from build123d import *

# Parameters (mm, degrees)
F0_W      = 2057.4
F0_H      = 1143
F1_DEPTH  = 19.05
F3_DEPTH  = 50.8
F5_DEPTH  = 50.8
F7_DEPTH  = 50.8
F10_DEPTH = 50.8
F12_DEPTH = 50.8
F14_DEPTH = 50.8
F16_DEPTH = 50.8
F18_DEPTH = 50.8


with BuildPart() as f1:
    # F0 (on Top) → F1 (new body)
    with BuildSketch(Plane.XY):
        Polygon((1066.8, 609.6), (0, 609.6), (-1066.8, 609.6), (-1066.8, -609.6), (-1028.7, -609.6), (1066.8, -609.6), align=None)
        Rectangle(F0_W, F0_H, mode=Mode.SUBTRACT)
        Rectangle(F0_W, F0_H)
    extrude(amount=F1_DEPTH)

    # F2 (on face) → F3 (join)
    with BuildSketch(Plane(origin=(0, 0, 0), x_dir=(1, 0, 0), z_dir=(0, 0, -1))):
        Polygon((-914.4, -457.2), (0, -457.2), (914.4, -457.2), (914.4, 457.2), (0, 457.2), (-914.4, 457.2), align=None)
        Polygon((895.35, -438.15), (0, -438.15), (-895.35, -438.15), (-895.35, 438.15), (0, 438.15), (895.35, 438.15), align=None, mode=Mode.SUBTRACT)
    extrude(amount=F3_DEPTH)

    # F4 (on face) → F5 (join)
    with BuildSketch(Plane(origin=(0, -438.15, 0), x_dir=(-1, 0, 0), z_dir=(0, 1, 0))):
        with BuildLine():
            Line((895.35, -762), (895.35, 0))
            Line((895.35, 0), (742.95, 0))
            Line((742.95, 0), (615.95, 0))
            ThreePointArc((615.95, 0), (705.7525612107, -37.1974387893), (742.95, -127))
            ThreePointArc((742.95, -127), (763.4615182258, -201.0530890645), (819.15, -254))
            ThreePointArc((819.15, -254), (837.8461266285, -276.4019366858), (844.55, -304.8))
            Line((844.55, -304.8), (844.55, -762))
            Line((844.55, -762), (895.35, -762))
        make_face()
    extrude(amount=F5_DEPTH)

    # F6 (on face) → F7 (join)
    with BuildSketch(Plane.XZ.offset(-438.15)):
        with BuildLine():
            Line((-742.95, 0), (-895.35, 0))
            Line((-895.35, 0), (-895.35, -127))
            Line((-895.35, -127), (-895.35, -203.2))
            Line((-895.35, -203.2), (-895.35, -762))
            Line((-895.35, -762), (-844.55, -762))
            Line((-844.55, -762), (-844.55, -304.8))
            ThreePointArc((-844.55, -304.8), (-837.8461266285, -276.4019366858), (-819.15, -254))
            ThreePointArc((-819.15, -254), (-760.8906614316, -202.595603141), (-742.95, -127))
            ThreePointArc((-742.95, -127), (-705.7525612107, -37.1974387893), (-615.95, 0))
            Line((-615.95, 0), (-742.95, 0))
        make_face()
    extrude(amount=F7_DEPTH)

    # F8: F1 across plane


with BuildPart() as f1_1:
    add(f1.part)
    add(f1.part.mirror(Plane.YZ))

    # F9 (on face) → F10 (join)
    with BuildSketch(Plane.XZ.offset(438.15)):
        with BuildLine():
            Line((-844.55, -558.8), (-844.55, -762))
            ThreePointArc((-844.55, -762), (0, -642.6582759858), (844.55, -762))
            Line((844.55, -762), (844.55, -558.8))
            Line((844.55, -558.8), (-844.55, -558.8))
        make_face()
    extrude(amount=-F10_DEPTH)

    # F11 (on face) → F12 (join)
    with BuildSketch(Plane(origin=(0, 438.15, 0), x_dir=(-1, 0, 0), z_dir=(0, 1, 0))):
        with BuildLine():
            ThreePointArc((-844.55, -762), (0, -642.6582759858), (844.55, -762))
            Line((844.55, -762), (844.55, -558.8))
            Line((844.55, -558.8), (-844.55, -558.8))
            Line((-844.55, -558.8), (-844.55, -762))
        make_face()
    extrude(amount=-F12_DEPTH)

    # F13 (on face) → F14 (join)
    with BuildSketch(Plane.YZ.offset(-895.35)):
        with BuildLine():
            Line((-387.35, -560.2836336464), (-387.35, -762))
            ThreePointArc((-387.35, -762), (0, -644.1417336464), (387.35, -762))
            Line((387.35, -762), (387.35, -560.2836336464))
            Line((387.35, -560.2836336464), (-387.35, -560.2836336464))
        make_face()
    extrude(amount=F14_DEPTH)

    # F15 (on face) → F16 (join)
    with BuildSketch(Plane(origin=(895.35, 0, 0), x_dir=(0, -1, 0), z_dir=(-1, 0, 0))):
        with BuildLine():
            Line((-387.35, -558.8), (-387.35, -762))
            ThreePointArc((-387.35, -762), (0, -642.6581), (387.35, -762))
            Line((387.35, -762), (387.35, -558.8))
            Line((387.35, -558.8), (-387.35, -558.8))
        make_face()
    extrude(amount=F16_DEPTH)

    # F17 (on face) → F18 (join)
    with BuildSketch(Plane.YZ.offset(-895.35)):
        with BuildLine():
            Line((387.35, -304.8), (387.35, 0))
            Line((387.35, 0), (158.75, 0))
            ThreePointArc((158.75, 0), (248.5525612107, -37.1974387893), (285.75, -127))
            ThreePointArc((285.75, -127), (306.2615182258, -201.0530890645), (361.95, -254))
            ThreePointArc((361.95, -254), (380.6461266285, -276.4019366858), (387.35, -304.8))
        make_face()
        with BuildLine():
            Line((-387.35, 0), (-387.35, -304.8))
            ThreePointArc((-387.35, -304.8), (-380.6461266285, -276.4019366858), (-361.95, -254))
            ThreePointArc((-361.95, -254), (-306.2615182258, -201.0530890645), (-285.75, -127))
            ThreePointArc((-285.75, -127), (-248.5525612107, -37.1974387893), (-158.75, 0))
            Line((-158.75, 0), (-387.35, 0))
        make_face()
    extrude(amount=F18_DEPTH)

    # F19: F1 across plane


with BuildPart() as f1_2:
    add(f1_1.part)
    add(f1_1.part.mirror(Plane.YZ))


solid = f1_2.part
The model under review builds one solid part; all positions refer to its coordinate system, in mm. A direction names the side the tool comes from. Round coordinates to 2 decimals unless told otherwise and drop trailing zeros. Order: outer loops, then holes, each group sorted by start corner. A loop starts at its lowest first (then second) coordinate and runs counter-clockwise, first axis right, second up. Notation, with made-up numbers: (-36, -16) -> (4, -16) arc R14 ccw to (4, -9) -> close; hole circle Ø11 at (60, 6). An arc over 180 degrees is marked (long way). Return JSON: item names as keys, results as strings.
1. Take a section at D-D (x = 499). Write out the cut boundary in (y, z), then the cut area to 3 significant figures.
Answer block:
{"outline": "(-609.6, 0) -> (-457.2, 0) -> (-457.2, -50.8) -> (-438.15, -50.8) -> (-438.15, 0) -> (438.15, 0) -> (438.15, -50.8) -> (457.2, -50.8) -> (457.2, 0) -> (609.6, 0) -> (609.6, 19.05) -> (-609.6, 19.05) -> close; (-438.15, -683.78) -> (-387.35, -683.78) -> (-387.35, -558.8) -> (-438.15, -558.8) -> close; (387.35, -683.78) -> (438.15, -683.78) -> (438.15, -558.8) -> (387.35, -558.8) -> close", "area": "37,900 mm²"}
2. Take a section at C-C (y = -229.5). Write out the cut boundary in (x, z).
Answer block:
{"outline": "(-1066.8, 0) -> (-914.4, 0) -> (-914.4, -50.8) -> (-895.35, -50.8) -> (-895.35, -21.53) -> (-844.55, -21.53) -> (-844.55, 0) -> (844.55, 0) -> (844.55, -21.53) -> (895.35, -21.53) -> (895.35, -50.8) -> (914.4, -50.8) -> (914.4, 0) -> (1066.8, 0) -> (1066.8, 19.05) -> (-1066.8, 19.05) -> close; (-895.35, -683.1) -> (-844.55, -683.1) -> (-844.55, -558.8) -> (-895.35, -558.8) -> close; (844.55, -683.1) -> (895.35, -683.1) -> (895.35, -558.8) -> (844.55, -558.8) -> close"}
3. For faces 1 (the face through (870, -5, -558.8)), 2 (the face through (12, 387.35, -614)), 3 (the face through (-706.735, 413.106, -38.19)), list the 3-axis set-ups (+Z, -Z, +X, -X, +Y, -Y) from which the entire face can be reached by the end or side of a thin tool; tool diameter is ignored.
Answer block:
{"face 1": "+X, -X", "face 2": "-Z", "face 3": "none"}
4. The part is to be moulded in two halves that separate along X. For faces 4 (the face through (-837.66, -413.11, -276.03)), 5 (the face through (-914.4, -6, -25)), 6 (the face through (-870.31, 380.46, -276.03)), 7 (the face through (-13, 6, 0)), say which applies: +X half, -X half, draft (parallel to the pull), parting line (faces both ways), or undercut.
Answer block:
{"face 4": "undercut", "face 5": "-X half", "face 6": "draft", "face 7": "undercut"}
5. Insertion check: P1, Ø15, axis at x = -286, z = -20, coming from the -Y side; P2, Ø6, axis at x = -466.5, y = 95, coming from the -Z side; P3, Ø15, axis at y = 402.5, z = -486, coming from the +X side. Each pin has a flat end and moves straight along its axis. Give the tip position at first contact, or say it passes through.
Answer block:
{"P1": "stops at y = -457.2", "P2": "stops at z = 0", "P3": "stops at x = 895.35"}
6. Take a section at A-A (x = -435.5). Write out the cut boundary in (y, z).
Answer block:
{"outline": "(-609.6, 0) -> (-457.2, 0) -> (-457.2, -50.8) -> (-438.15, -50.8) -> (-438.15, 0) -> (438.15, 0) -> (438.15, -50.8) -> (457.2, -50.8) -> (457.2, 0) -> (609.6, 0) -> (609.6, 19.05) -> (-609.6, 19.05) -> close; (-438.15, -673.93) -> (-387.35, -673.93) -> (-387.35, -558.8) -> (-438.15, -558.8) -> close; (387.35, -673.93) -> (438.15, -673.93) -> (438.15, -558.8) -> (387.35, -558.8) -> close"}
7. Take a section at B-B (z = -192.5). Write out the cut boundary in (x, y), then the cut area to 3 significant figures.
Answer block:
{"outline": "(-895.35, -438.15) -> (-758.72, -438.15) -> (-758.72, -387.35) -> (-844.55, -387.35) -> (-844.55, -301.52) -> (-895.35, -301.52) -> close; (-895.35, 301.52) -> (-844.55, 301.52) -> (-844.55, 387.35) -> (-755.43, 387.35) -> (-755.43, 438.15) -> (-895.35, 438.15) -> close; (755.43, 387.35) -> (844.55, 387.35) -> (844.55, 301.52) -> (895.35, 301.52) -> (895.35, 438.15) -> (755.43, 438.15) -> close; (758.72, -438.15) -> (895.35, -438.15) -> (895.35, -301.52) -> (844.55, -301.52) -> (844.55, -387.35) -> (758.72, -387.35) -> close", "area": "45,500 mm²"}
8. For L1, parallel to X at y = -381, z = -170; L2, parallel to Y at x = 380, z = -571, list the stretches that pass through material, from the lowest coordinate up. Write a range as [from, to].
Answer block:
{"L1": "x = [-895.35, -844.55], [844.55, 895.35]", "L2": "y = [-438.15, -387.35], [387.35, 438.15]"}
